Verification items for the finished model (mm, model axes). Face numbers are marked on the shaded views. Round coordinates to 2 decimals unless told otherwise and drop trailing zeros. Loops run counter-clockwise (first coordinate to the right, second up) from the corner with the lowest first, then second, coordinate; pieces in that order, holes last. Notation, with made-up numbers: M 44.25,88 L 100.25,88 A27 cw 100.25,122 Z; hole C 7.25,36.25 d5. An arc over 180 degrees is marked long. One line per item, written item: value.
from build123d import *

# Parameters (mm, degrees)
F0_R     = 2.5
F1_DEPTH = 5
F2_R     = 0.1


with BuildPart() as f1:
    # F0 (on Top) → F1 (new body)
    with BuildSketch(Plane.XY):
        Polygon((5.773503, 0), (2.886751, 5), (-2.886751, 5), (-5.773503, 0), (-2.886751, -5), (2.886751, -5), align=None)
        Circle(F0_R, mode=Mode.SUBTRACT)
    extrude(amount=F1_DEPTH)

    # F2
    f2_edges = [f1.edges().sort_by_distance(p)[0] for p in [
        (-2.886751, -5, 2.5),
        (2.886751, -5, 2.5),
        (0, -5, 0),
        (0, -5, 5),
        (-5.773503, 0, 2.5),
        (-4.330127, -2.5, 0),
        (-4.330127, -2.5, 5),
        (5.773503, 0, 2.5),
        (4.330127, -2.5, 0),
        (4.330127, -2.5, 5),
        (2.886751, 5, 2.5),
        (4.330127, 2.5, 0),
        (4.330127, 2.5, 5),
        (-2.886751, 5, 2.5),
        (0, 5, 0),
        (0, 5, 5),
        (-4.330127, 2.5, 0),
        (-4.330127, 2.5, 5),
        (-2.5, 0, 5),
    ]]
    fillet(f2_edges, radius=F2_R)


solid = f1.part
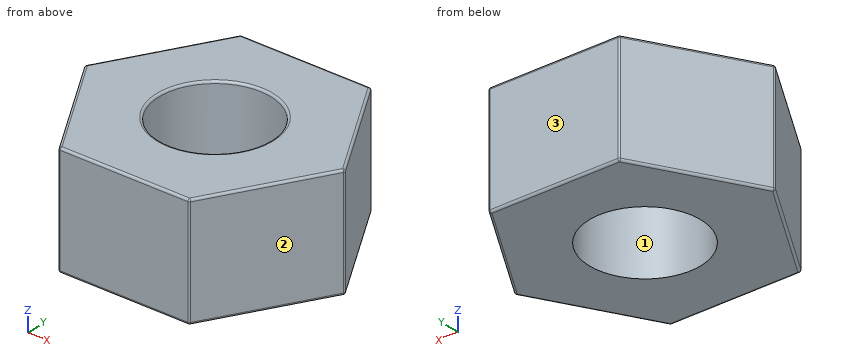
(1) Thickness scan on L1, parallel to Y at x = 0, z = 2.2; L2, parallel to X at y = -2, z = 4.1; L3, parallel to X at y = -0.75, z = 2.6. Record the ranges inside material, lowest first. Write a range as from..to.
Completed:
L1: y = -5..-2.5, 2.5..5
L2: x = -4.62..-1.5, 1.5..4.62
L3: x = -5.34..-2.38, 2.38..5.34
(2) Depth check by flat-ended pin: pin 1 Ø1 at (y, z) = (2.5, 3.5) entering from +X; pin 2 Ø2 at (x, z) = (4, 4) entering from +Y. Enter the tip coordinate at first touch or a pass-through.
Completed:
pin 1: stops at x = 4.62
pin 2: stops at y = 4.8
(3) Sectioned sample at B-B on z = 2.6. Enter the section's corners in (x, y), and give its area (3 significant figures).
Completed:
outline: M -5.74,-0.05 L -2.92,-4.95 A0.1 ccw -2.83,-5 L 2.83,-5 A0.1 ccw 2.92,-4.95 L 5.74,-0.05 A0.1 ccw 5.74,0.05 L 2.92,4.95 A0.1 ccw 2.83,5 L -2.83,5 A0.1 ccw -2.92,4.95 L -5.74,0.05 A0.1 ccw Z; hole C 0,0 d5
area: 67.0 mm^2
(4) Mould release check, pull along Y, two halves, no side actions. Record for the marked faces 1, 2 and 3: +Y half, -Y half, draft (parallel to the pull), parting line (faces both ways), or undercut.
Completed:
face 1: undercut
face 2: -Y half
face 3: +Y half
(5) Sectioned sample at A-A on x = 0. Enter the section's corners in (y, z).
Completed:
outline: M -5,0.1 A0.1 ccw -4.9,0 L -2.5,0 L -2.5,4.9 A0.1 ccw -2.6,5 L -4.9,5 A0.1 ccw -5,4.9 Z; M 2.5,0 L 4.9,0 A0.1 ccw 5,0.1 L 5,4.9 A0.1 ccw 4.9,5 L 2.6,5 A0.1 ccw 2.5,4.9 Z
